Geometry: final body of the model. Coordinates: model frame, mm. Give positions to 0.01 mm unless a question says otherwise; leave off trailing zeros. Order: outer loops, then holes, each group sorted by start corner. A loop starts at its lowest first (then second) coordinate and runs counter-clockwise, first axis right, second up. Notation, with made-up numbers: (-22, -4) -> (-16, -4) arc R14 ccw to (-16, 15) -> close; hole circle Ø3 at (14.25, -16). An arc over 180 degrees is marked (long way). One line per question, with ' | ' between items.
from build123d import *

# Parameters (mm, degrees)
EXTRUDE_1_DEPTH     = 4
SKETCH_2_R          = 2.5
CUT_EXTRUDE_1_DEPTH = 4
FILLET_1_R          = 0.1


with BuildPart() as part:
    # 草图1 → 凸台-拉伸1 (new body)
    with BuildSketch(Plane.XY):
        Polygon((0, 4.618802154), (-4, 2.309401077), (-4, -2.309401077), (0, -4.618802154), (4, -2.309401077), (4, 2.309401077), align=None)
    extrude(amount=EXTRUDE_1_DEPTH)

    # 草图2 → 切除-拉伸1 (cut)
    with BuildSketch(Plane.XY.offset(4)):
        Circle(SKETCH_2_R)
    extrude(amount=-CUT_EXTRUDE_1_DEPTH, mode=Mode.SUBTRACT)

    # 圆角1
    fillet_1_edges = [part.edges().sort_by_distance(p)[0] for p in [
        (-2.5, 0, 0),
    ]]
    fillet(fillet_1_edges, radius=FILLET_1_R)

    # 草图3 → 切除-旋转2 (revolve, cut)
    with BuildSketch(Plane(origin=(0, 0, 0), x_dir=(0, 0, -1), z_dir=(1, 0, 0))):
        Polygon((0, 4.618802154), (0, 3.998802154), (-0.62, 4.618802154), align=None)
        Polygon((-3.38, 4.618802154), (-4, 3.998802154), (-4, 4.618802154), align=None)
    revolve(axis=Axis((0, 0, 0), (0, 0, -1)), mode=Mode.SUBTRACT)


solid = part.part
1) Contact query for flat-ended pins moving along their axis: pin 1 Ø4.5 at (x, y) = (0, 0) entering from -Z; pin 2 Ø2 at (y, z) = (3, 3) entering from +X. Output: stop coordinate, or through.
Check result:
pin 1: passes through | pin 2: stops at x = 4
2) Material intervals for probe 1 along Y at (x, z) = (-0.5, 1.7); probe 2 along Y at (x, z) = (-1, 2.4); probe 3 along X at (y, z) = (2, 2.05), sorted ascending. Write a range as from..to.
Check result:
probe 1: y = -4.33..-2.45, 2.45..4.33 | probe 2: y = -4.04..-2.29, 2.29..4.04 | probe 3: x = -4..-1.5, 1.5..4
3) Section B-B on z = 1.3. Return loops of the section in (x, y).
Check result:
outline: (-4, -2.31) -> (0, -4.62) -> (4, -2.31) -> (4, 2.31) -> (0, 4.62) -> (-4, 2.31) -> close; hole circle Ø5 at (0, 0)
4) Pull-direction query (Y, two-part tool) for faces 1 (the cylindrical face through (-0.54, -2.44, 2.08)), 2 (the flat face through (1.97, -3.48, 1.97)), 3 (the flat face through (-4, 0, 2)); classes: +Y half, -Y half, draft (parallel to the pull), parting line (faces both ways), or undercut.
Check result:
face 1: undercut | face 2: -Y half | face 3: draft
